Geometry check sheet. Reference: the model listing, model coordinates, mm. Face numbers are marked on the shaded views. A direction names the side the tool comes from. Round coordinates to 2 decimals unless told otherwise and drop trailing zeros. Order: outer loops, then holes, each group sorted by start corner. A loop starts at its lowest first (then second) coordinate and runs counter-clockwise, first axis right, second up. Notation, with made-up numbers: (2, -13.75) - (40, -13.75) arc R23 ccw to (40, -4.75) - close; hole circle Ø7 at (53.5, 1). An arc over 180 degrees is marked (long way). Use a Markdown table: item, result. Add a question column.
(1) Section check C-C on y = -0.5. Record the boundary of the cut face in (x, z), then the cut area to 3 significant figures.
(2) Gauge pin test, flat ends, axial feed: P1, Ø2, axis at x = -1.5, y = -1, coming from the -Z side; P2, Ø3.5, axis at x = 0, z = 36.5, coming from the -Y side. Record the tip position at first contact, or that the pin passes through.
(3) Mould release check, pull along X, two halves, no side actions. Record for the marked faces 3, 4 and 5: released by +X, released by -X, zero draft, split by the parting line, or undercut.
(4) Access from +Z, -Z, +X, -X, +Y, -Y to the whole of each face (thin tool, end or side, straight path). Record for the marked faces 1 and 2.
(5) Section check A-A on z = 36.5. Record the boundary of the cut face in (x, y), then the cut area to 3 significant figures.
(6) Section check B-B on x = 0. Record the boundary of the cut face in (y, z).
(7) Thickness scan on line 1 along Z through (x, y) = (0, -4.2); line 2 along X through (y, z) = (-4.2, 3.5); line 3 along Y through (x, z) = (-0.5, 5). Record the ranges inside material, lowest first. Write a range as [from, to].
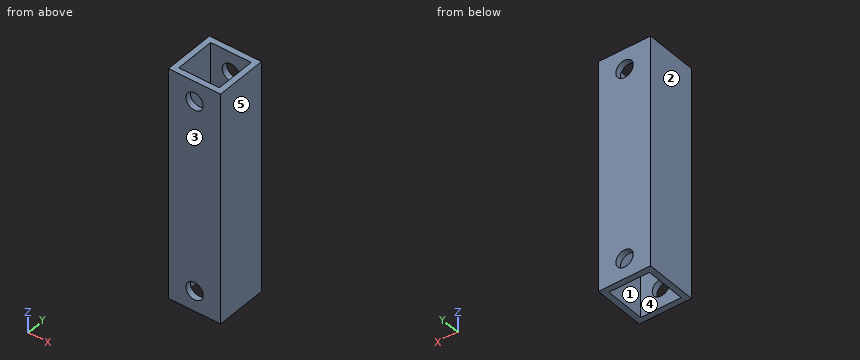
```python
from build123d import *

# Parameters (mm, degrees)
SKETCH_1_W          = 9
SKETCH_1_H          = 9
EXTRUDE_1_DEPTH     = 40
SKETCH_2_W          = 7
SKETCH_2_H          = 7
CUT_EXTRUDE_1_DEPTH = 40
SKETCH_3_R          = 1.5
CUT_EXTRUDE_2_DEPTH = 38


with BuildPart() as part:
    # ｽｹｯﾁ1 → ﾎﾞｽ - 押し出し1 (new body)
    with BuildSketch(Plane.XY):
        Rectangle(SKETCH_1_W, SKETCH_1_H)
    extrude(amount=EXTRUDE_1_DEPTH)

    # ｽｹｯﾁ2 → ｶｯﾄ - 押し出し1 (cut)
    with BuildSketch(Plane.XY.offset(40)):
        Rectangle(SKETCH_2_W, SKETCH_2_H)
    extrude(amount=-CUT_EXTRUDE_1_DEPTH, mode=Mode.SUBTRACT)

    # ｽｹｯﾁ3 → ｶｯﾄ - 押し出し2 (cut)
    with BuildSketch(Plane(origin=(0, 4.5, 0), x_dir=(1, 0, 0), z_dir=(0, 1, 0))):
        with Locations((0, -3.5)):
            Circle(SKETCH_3_R)
        with Locations((0, -36.5)):
            Circle(SKETCH_3_R)
    extrude(amount=-CUT_EXTRUDE_2_DEPTH, mode=Mode.SUBTRACT)


solid = part.part
```
Check sheet entries:
| question | item | result |
|---|---|---|
| 1 | outline | (-4.5, 0) - (-3.5, 0) - (-3.5, 40) - (-4.5, 40) - close; (3.5, 0) - (4.5, 0) - (4.5, 40) - (3.5, 40) - close |
| 1 | area | 80.0 mm2 |
| 2 | P1 | passes through |
| 2 | P2 | stops at y = -4.5 |
| 3 | face 3 | zero draft |
| 3 | face 4 | undercut |
| 3 | face 5 | released by +X |
| 4 | face 1 | +Z, -Z |
| 4 | face 2 | +Z, -Z, -X, +Y, -Y |
| 5 | outline | (-4.5, -4.5) - (-1.5, -4.5) - (-1.5, -3.5) - (-3.5, -3.5) - (-3.5, 3.5) - (-1.5, 3.5) - (-1.5, 4.5) - (-4.5, 4.5) - close; (1.5, -4.5) - (4.5, -4.5) - (4.5, 4.5) - (1.5, 4.5) - (1.5, 3.5) - (3.5, 3.5) - (3.5, -3.5) - (1.5, -3.5) - close |
| 5 | area | 26.0 mm2 |
| 6 | outline | (-4.5, 0) - (-3.5, 0) - (-3.5, 2) - (-4.5, 2) - close; (-4.5, 5) - (-3.5, 5) - (-3.5, 35) - (-4.5, 35) - close; (-4.5, 38) - (-3.5, 38) - (-3.5, 40) - (-4.5, 40) - close; (3.5, 0) - (4.5, 0) - (4.5, 2) - (3.5, 2) - close; (3.5, 5) - (4.5, 5) - (4.5, 35) - (3.5, 35) - close; (3.5, 38) - (4.5, 38) - (4.5, 40) - (3.5, 40) - close |
| 7 | line 1 | z = [0, 2], [5, 35], [38, 40] |
| 7 | line 2 | x = [-4.5, -1.5], [1.5, 4.5] |
| 7 | line 3 | y = [-4.5, -3.5], [3.5, 4.5] |
